Part model, mm, in its own coordinate system. Round coordinates to 2 decimals unless told otherwise and drop trailing zeros. Write each loop counter-clockwise with the first axis right and the second up, starting at its lowest first coordinate (ties: lowest second). Pieces come first, ordered by that corner, then holes. Notation, with made-up numbers: M -27,21.5 L 5,21.5 A14 cw 5,44.5 Z; hole C -16.75,-32.75 d7. An arc over 180 degrees is marked long. Use a Markdown table: item, result. Add a question column.
1) Drop flat-ended pins along their axis: P1, Ø5.5, axis at x = -57.15, y = 31.75, coming from the -Z side; P2, Ø4, axis at y = 72, z = -8, coming from the +X side; P3, Ø3.5, axis at x = -171.45, y = 31.75, coming from the -Z side; P4, Ø1, axis at y = 35, z = -8, coming from the +X side. Give the stop position or say it passes through.
2) Slice it at B-B on x = -171.45. Write the cut outline in (y, z).
3) Slice it at C-C on y = 31.75. Give the number of separate pieces and of enclosed holes in the cut face, plus the area to 3 significant figures.
4) Wall check: probe 1 along Y at (x, z) = (-69.85, 1.05); probe 2 along Y at (x, z) = (-171.45, 0.75); probe 3 along Z at (x, y) = (-84, 83). Give the ranges that are in metal, low to high.
5) Two-plate mould, pull along X, no slides. Class faces 1 (the face through (-173.183, 30.421, 0.805)), 2 (the face through (-190.79, 51.51, -5.05)), 3 (the face through (-93, 52, 0)): released by +X, released by -X, zero draft, split by the parting line, or undercut.
Autodesk Inventor part; units mm, degrees
ref_plane "YZ Plane" through (0, 0, 0) normal (1, 0, 0) x (0, 1, 0)
ref_plane "XZ Plane" through (0, 0, 0) normal (0, 1, 0) x (-1, 0, 0)
ref_plane "XY Plane" through (0, 0, 0) normal (0, 0, 1) x (1, 0, 0)
sketch "Sketch1" plane through (0, 0, 0) normal (0, 0, 1) x (1, 0, 0)
  line L0 (0, 0) -> (-184.15, 0)
  line L1 (-184.15, 0) -> (-184.15, 101.6)
  line L2 (-184.15, 101.6) -> (0, 101.6)
  line L3 (0, 101.6) -> (0, 0)
  dimension "d0" = 184.15
  dimension "d1" = 101.6
extrude "Extrusion1" add sketch "Sketch1" along normal blind 1.5875
chamfer "Chamfer1" distance 1.5875 angle 45 1 edges at (-184.15, 50.8, 0)
sketch "Sketch2" plane through (-184.15, 0, 1.5875) normal (-0.7071, 0, -0.7071) x (-0.7071, 0, 0.7071)
  line L0 (0, 101.6) -> (0, 0)
  line L1 (-2.2451, 101.6) -> (-2.2451, 0)
  line L2 (0, 101.6) -> (-2.2451, 101.6)
  line L3 (-2.2451, 0) -> (0, 0)
  point P0 (-131.3362, 0)
extrude "Extrusion2" add sketch "Sketch2" along normal blind 19.05
sketch "Sketch3" plane through (0, 0, 1.5875) normal (0, 0, 1) x (1, 0, 0)
  circle A0 centre (-57.15, 31.75) radius 2.1844
  line L0 (-184.15, 0) -> (0, 0)
  line L1 (-184.15, 101.6) -> (-184.15, 0)
  circle A1 centre (-69.85, 44.45) radius 2.1844
  circle A2 centre (-171.45, 31.75) radius 2.1844
  point P0 (-231.8428, 57.2075)
  dimension "d9" = 4.3688
  dimension "d10" = 31.75
  dimension "d11" = 127
  dimension "d12" = 4.3688
  dimension "d13" = 44.45
  dimension "d14" = 114.3
  dimension "d17" = 4.3688
  dimension "d18" = 114.3
extrude "Extrusion3" cut sketch "Sketch3" against normal blind 19.05
properties part number "frontwing"
Entries:
| question | item | result |
|---|---|---|
| 1 | P1 | stops at z = 0 |
| 1 | P2 | stops at x = -188.56 |
| 1 | P3 | passes through |
| 1 | P4 | stops at x = -190.06 |
| 2 | outline | M 0,0 L 29.57,0 L 29.57,1.59 L 0,1.59 Z; M 33.93,0 L 101.6,0 L 101.6,1.59 L 33.93,1.59 Z |
| 3 | separate pieces | 3 |
| 3 | enclosed holes | 0 |
| 3 | area | 320 mm^2 |
| 4 | probe 1 | y = 0 to 42.27, 46.63 to 101.6 |
| 4 | probe 2 | y = 0 to 29.57, 33.93 to 101.6 |
| 4 | probe 3 | z = 0 to 1.59 |
| 5 | face 1 | undercut |
| 5 | face 2 | released by -X |
| 5 | face 3 | zero draft |
